Verification items for the finished model (mm, model axes). A direction names the side the tool comes from. Round coordinates to 2 decimals unless told otherwise and drop trailing zeros. Write each loop counter-clockwise with the first axis right and the second up, starting at its lowest first coordinate (ties: lowest second). Pieces come first, ordered by that corner, then holes. Notation, with made-up numbers: M 60,3 L 93,3 A31 ccw 93,30 Z; hole C 9.25,-4 d2. An arc over 180 degrees is marked long. One line per item, written item: value. Start each with the question number.
Item 1: Section check A-A, the plane x = 0. Record the cut outline in (y, z) (3 decimals), then the cut area to 3 significant figures.
Item 2: Tool access check on faces 1 (the face through (0, -6, -3)), 2 (the face through (-2.4, 0, 3)), 3 (the face through (6, -11, 3)). Record the directions out of +Z, -Z, +X, -X, +Y, -Y that give a thin tool (end or side, any length) a straight path to the whole face; none if there is none.
Item 3: Section check C-C, the plane z = 6.25. Record the cut outline in (x, y) (3 decimals).
Item 4: Draft check along X on faces 4 (the face through (3, -2, 9)), 5 (the face through (-7.559, -5.796, 5.986)), 6 (the face through (11.356, -23.102, -0.042)). Enter one of: +X half, -X half, draft (parallel to the pull), parting line (faces both ways), or undercut.
Item 5: Gauge pin test, flat ends, axial feed: pin 1 (1.5 mm diameter, centred on x = 14.5, y = -1, fed in from +Z); pin 2 (2 mm diameter, centred on x = -15, z = 0, fed in from +Y); pin 3 (1 mm diameter, centred on x = 18, z = 1, fed in from +Y); pin 4 (4.5 mm diameter, centred on x = 23.81, y = 0, fed in from -Z). Record the tip position at first contact, or that the pin passes through.
Item 6: Thickness scan on probe 1 along X at (y, z) = (20.5, 0.5); probe 2 along Z at (x, y) = (-6, 16); probe 3 along X at (y, z) = (-2, 4.25). Record the ranges inside material, lowest first. Write a range as from..to.
Item 7: Section check B-B, the plane z = -1.25. State how many separate pieces and enclosed holes the cut face has, then the cut area to 3 significant figures.
from build123d import *

# Parameters (mm, degrees)
SKETCH1_R           = 28.575
SKETCH1_R_2         = 2.54
BOSS_EXTRUDE1_DEPTH = 3
SKETCH2_R           = 9.525
BOSS_EXTRUDE2_DEPTH = 6
CUT_EXTRUDE1_REACH  = 44.155
FILLET1_R           = 2


with BuildPart() as part:
    # Sketch1 → Boss-Extrude1 (new, symmetric)
    with BuildSketch(Plane.XY):
        Circle(SKETCH1_R)
        with Locations((-23.8125, 0)):
            Circle(SKETCH1_R_2, mode=Mode.SUBTRACT)
        with Locations((-11.90625, 20.622229928)):
            Circle(SKETCH1_R_2, mode=Mode.SUBTRACT)
        with Locations((11.90625, 20.622229928)):
            Circle(SKETCH1_R_2, mode=Mode.SUBTRACT)
        with Locations((23.8125, 0)):
            Circle(SKETCH1_R_2, mode=Mode.SUBTRACT)
        with Locations((11.90625, -20.622229928)):
            Circle(SKETCH1_R_2, mode=Mode.SUBTRACT)
        with Locations((-11.90625, -20.622229928)):
            Circle(SKETCH1_R_2, mode=Mode.SUBTRACT)
    extrude(amount=BOSS_EXTRUDE1_DEPTH, both=True)

    # Sketch2 → Boss-Extrude2 (add)
    with BuildSketch(Plane.XY.offset(3)):
        Circle(SKETCH2_R)
    extrude(amount=BOSS_EXTRUDE2_DEPTH)

    # Sketch3 → Cut-Extrude1 (cut, up to next)
    with BuildSketch(Plane.XY.offset(9), mode=Mode.PRIVATE) as cut_extrude1_sk1:
        with BuildLine():
            ThreePointArc((3.3, 0), (1.218605761, 3.066757245), (-2.4, 2.264950331))
            Line((-2.4, 2.264950331), (-2.4, -2.264950331))
            ThreePointArc((-2.4, -2.264950331), (1.218605761, -3.066757245), (3.3, 0))
        make_face()
    cut_extrude1_tool1 = extrude(cut_extrude1_sk1.sketch, amount=-CUT_EXTRUDE1_REACH, mode=Mode.PRIVATE) & part.part
    add(cut_extrude1_tool1.solids().sort_by_distance((0.246613, 0, 9))[0], mode=Mode.SUBTRACT)

    # Fillet1
    fillet1_edges = [part.edges().sort_by_distance(p)[0] for p in [
        (-9.525, 0, 3),
        (-9.525, 0, 9),
        (-28.575, 0, 3),
    ]]
    fillet(fillet1_edges, radius=FILLET1_R)


solid = part.part
Response values:
1. outline: M -28.575,-3 L -3.3,-3 L -3.3,9 L -7.525,9 A2 ccw -9.525,7 L -9.525,5 A2 cw -11.525,3 L -26.575,3 A2 ccw -28.575,1 Z; M 3.3,-3 L 28.575,-3 L 28.575,1 A2 ccw 26.575,3 L 11.525,3 A2 cw 9.525,5 L 9.525,7 A2 ccw 7.525,9 L 3.3,9 Z
1. area: 376 mm2
2. face 1: -Z, +X, -X, +Y, -Y
2. face 2: +Z, -Z
2. face 3: +Z
3. outline: C 0,0 d19.05; hole M -2.4,-2.265 A3.3 ccw long -2.4,2.265 Z
4. face 4: draft
4. face 5: parting line
4. face 6: undercut
5. pin 1: stops at z = 3
5. pin 2: stops at y = 24.91
5. pin 3: stops at y = 22.59
5. pin 4: passes through
6. probe 1: x = -19.91..-14.44, -9.37..9.37, 14.44..19.91
6. probe 2: z = -3..3
6. probe 3: x = -9.46..-2.4, 2.62..9.46
7. separate pieces: 1
7. enclosed holes: 7
7. area: 2,410 mm2
